The listing builds one solid part. Answer for the finished solid, in the listing's coordinates (mm). A direction names the side the tool comes from. Coordinates: 2 decimals unless noted, no trailing zeros. Write each loop counter-clockwise with the first axis right and the second up, starting at its lowest first coordinate (ties: lowest second). Pieces come first, ordered by that corner, then holes.
(1) Straight lines are drawn through the part: line 1 (X direction, y = -2.5, z = -21.5); line 2 (X direction, y = -17, z = 30.5); line 3 (Z direction, x = 26, y = -11). For each, find the intervals that lie inside material, in ascending order.
(2) The part is cut by section A-A on y = -11. Determine the outline of the cut face in (x, z).
(3) The part is cut by section D-D on z = 13. Determine the outline of the cut face in (x, y), plus the area to 3 significant figures.
(4) The part is cut by section C-C on z = 32.5. Determine the outline of the cut face in (x, y), plus the area to 3 significant figures.
(5) The part is cut by section B-B on x = 11.5. Determine the outline of the cut face in (y, z), plus the area to 3 significant figures.
(6) Which of the six approach directions +Z, -Z, +X, -X, +Y, -Y give full straight-line access (tool end or side, diameter ignored) to faces 1 (the cylindrical face through (4.888, 3.402, 28.834)), 2 (the cylindrical face through (9.86, 1.43, 45.14)), 3 (the flat face through (23, -8, 16)), 4 (the cylindrical face through (26.41, 9.71, 57.75))?
(7) For a pull along Y with two mould halves and no side action, classify faces 5 (the flat face through (23, 7, -28.402)), 6 (the cylindrical face through (-2.43, 23.376, 15.517)), 7 (the cylindrical face through (-1.479, -3.464, 33.028)) as +Y half, -Y half, draft (parallel to the pull), parting line (faces both ways), or undercut.
(8) Given P1, Ø1.5, axis at x = 16.5, z = 42.5, coming from the -Y side; P2, Ø6, axis at x = 24, z = 42, coming from the +Y side; P3, Ø10, axis at x = 11, z = 26.5, coming from the -Y side, each flat-ended and moving along its own axis, determine where each tip first touches the part or whether it passes through.
from build123d import *

# Parameters (mm, degrees)
RESSALTO_EXTRUS_O2_DEPTH      = 30
RESSALTO_EXTRUS_O3_DEPTH      = 3
RESSALTO_EXTRUS_O4_DEPTH      = 3
RESSALTO_EXTRUS_O4_DEPTH_BACK = 10
CORTE_EXTRUS_O1_DEPTH         = 10
CORTE_EXTRUS_O2_DEPTH         = 23.75
ESBO_O10_R                    = 1.5
CORTE_EXTRUS_O3_DEPTH         = 10
CORTE_EXTRUS_O4_DEPTH         = 10
FILETE2_R                     = 2
ESBO_O13_R                    = 1.5
CORTE_EXTRUS_O5_DEPTH         = 16
CORTE_EXTRUS_O11_DEPTH        = 117
FILETE7_R                     = 6
ESBO_O18_R                    = 4
CORTE_EXTRUS_O13_DEPTH        = 22
ESBO_O19_R                    = 4
CORTE_EXTRUS_O14_DEPTH        = 22


with BuildPart() as part:
    # Esboço2 → Ressalto-extrusão2 (new body)
    with BuildSketch(Plane(origin=(0, 0, 0), x_dir=(0, 0, -1), z_dir=(1, 0, 0))):
        with BuildLine():
            Line((2.90159992, -0.062465938), (-35.09840008, -0.062465938))
            Line((-35.09840008, -0.062465938), (-39.886084903, -0.062465938))
            ThreePointArc((-39.886084903, -0.062465938), (-45.202180234, 1.467638524), (-48.891439328, 5.589707975))
            ThreePointArc((-48.891439328, 5.589707975), (-52.096536948, 9.772081499), (-56.69840008, 12.338743681))
            ThreePointArc((-56.69840008, 12.338743681), (-59.373224015, 11.895603401), (-60.59840008, 9.476926077))
            Line((-60.59840008, 9.476926077), (-60.59840008, 20.976926077))
            ThreePointArc((-60.59840008, 20.976926077), (-59.719720424, 23.09824642), (-57.59840008, 23.976926077))
            Line((-57.59840008, 23.976926077), (25.40159992, 23.976926077))
            ThreePointArc((25.40159992, 23.976926077), (27.522920263, 23.09824642), (28.40159992, 20.976926077))
            Line((28.40159992, 20.976926077), (28.40159992, 9.476926077))
            ThreePointArc((28.40159992, 9.476926077), (27.176423855, 11.895603401), (24.50159992, 12.338743681))
            ThreePointArc((24.50159992, 12.338743681), (19.899736788, 9.772081499), (16.694639168, 5.589707975))
            ThreePointArc((16.694639168, 5.589707975), (13.005380073, 1.467638524), (7.689284743, -0.062465938))
            Line((7.689284743, -0.062465938), (2.90159992, -0.062465938))
        make_face()
    extrude(amount=RESSALTO_EXTRUS_O2_DEPTH)

    # Esboço3 → Ressalto-extrusão3 (add)
    with BuildSketch(Plane.ZY):
        with BuildLine():
            Line((60.59840008, 15.226926077), (60.59840008, 20.976926077))
            ThreePointArc((60.59840008, 20.976926077), (59.719720424, 23.09824642), (57.59840008, 23.976926077))
            Line((57.59840008, 23.976926077), (16.09840008, 23.976926077))
            Line((16.09840008, 23.976926077), (-25.40159992, 23.976926077))
            ThreePointArc((-25.40159992, 23.976926077), (-27.522920263, 23.09824642), (-28.40159992, 20.976926077))
            Line((-28.40159992, 20.976926077), (-28.40159992, 15.226926077))
            Line((-28.40159992, 15.226926077), (-28.40159992, -16.773073923))
            ThreePointArc((-28.40159992, -16.773073923), (-27.522920263, -18.894394267), (-25.40159992, -19.773073923))
            Line((-25.40159992, -19.773073923), (57.59840008, -19.773073923))
            ThreePointArc((57.59840008, -19.773073923), (59.719720424, -18.894394267), (60.59840008, -16.773073923))
            Line((60.59840008, -16.773073923), (60.59840008, 15.226926077))
        make_face()
    extrude(amount=RESSALTO_EXTRUS_O3_DEPTH)

    # Esboço4 → Ressalto-extrusão4 (add, two sides)
    with BuildSketch(Plane(origin=(30, 0, 0), x_dir=(0, 0, -1), z_dir=(1, 0, 0))) as ressalto_extrus_o4_sk:
        with BuildLine():
            Line((-16.09840008, 23.976926077), (25.40159992, 23.976926077))
            ThreePointArc((25.40159992, 23.976926077), (27.522920263, 23.09824642), (28.40159992, 20.976926077))
            Line((28.40159992, 20.976926077), (28.40159992, 15.226926077))
            Line((28.40159992, 15.226926077), (28.40159992, -16.773073923))
            ThreePointArc((28.40159992, -16.773073923), (27.522920263, -18.894394267), (25.40159992, -19.773073923))
            Line((25.40159992, -19.773073923), (-57.59840008, -19.773073923))
            ThreePointArc((-57.59840008, -19.773073923), (-59.719720424, -18.894394267), (-60.59840008, -16.773073923))
            Line((-60.59840008, -16.773073923), (-60.59840008, 15.226926077))
            Line((-60.59840008, 15.226926077), (-60.59840008, 20.976926077))
            ThreePointArc((-60.59840008, 20.976926077), (-59.719720424, 23.09824642), (-57.59840008, 23.976926077))
            Line((-57.59840008, 23.976926077), (-16.09840008, 23.976926077))
        make_face()
    extrude(amount=RESSALTO_EXTRUS_O4_DEPTH)
    extrude(ressalto_extrus_o4_sk.sketch, amount=-RESSALTO_EXTRUS_O4_DEPTH_BACK)

    # Esboço8 → Corte-extrusão1 (cut)
    with BuildSketch(Plane(origin=(33, 0, 0), x_dir=(0, 0, -1), z_dir=(1, 0, 0))):
        with BuildLine():
            Line((-43.59840008, 3.976926077), (11.40159992, 3.976926077))
            ThreePointArc((11.40159992, 3.976926077), (12.815813482, 3.391139639), (13.40159992, 1.976926077))
            Line((13.40159992, 1.976926077), (13.40159992, -7.773073923))
            Line((13.40159992, -7.773073923), (13.40159992, -19.773073923))
            Line((13.40159992, -19.773073923), (-45.59840008, -19.773073923))
            Line((-45.59840008, -19.773073923), (-45.59840008, -7.773073923))
            Line((-45.59840008, -7.773073923), (-45.59840008, 1.976926077))
            ThreePointArc((-45.59840008, 1.976926077), (-45.012613643, 3.391139639), (-43.59840008, 3.976926077))
        make_face()
    extrude(amount=-CORTE_EXTRUS_O1_DEPTH, mode=Mode.SUBTRACT)

    # Esboço9 → Corte-extrusão2 (cut)
    with BuildSketch(Plane(origin=(0, -19.773073923, 0), x_dir=(-1, 0, 0), z_dir=(0, -1, 0))):
        with BuildLine():
            Line((-25, 13.40159992), (-28, 13.40159992))
            ThreePointArc((-28, 13.40159992), (-29.414213562, 12.815813482), (-30, 11.40159992))
            Line((-30, 11.40159992), (-30, -43.59840008))
            ThreePointArc((-30, -43.59840008), (-29.414213562, -45.012613643), (-28, -45.59840008))
            Line((-28, -45.59840008), (-25, -45.59840008))
            ThreePointArc((-25, -45.59840008), (-23.585786438, -45.012613643), (-23, -43.59840008))
            Line((-23, -43.59840008), (-23, 11.40159992))
            ThreePointArc((-23, 11.40159992), (-23.585786438, 12.815813482), (-25, 13.40159992))
        make_face()
    extrude(amount=-CORTE_EXTRUS_O2_DEPTH, mode=Mode.SUBTRACT)

    # Esboço10 → Corte-extrusão3 (cut)
    with BuildSketch(Plane(origin=(0, 0, 0), x_dir=(0, 0, -1), z_dir=(1, 0, 0))):
        with Locations((-55.59840008, 6.338743681)):
            Circle(ESBO_O10_R)
        with Locations((23.40159992, 6.338743681)):
            Circle(ESBO_O10_R)
        with Locations((-16.09840008, -8.562465938)):
            Circle(ESBO_O10_R)
    extrude(amount=-CORTE_EXTRUS_O3_DEPTH, mode=Mode.SUBTRACT)

    # Esboço12 → Corte-extrusão4 (cut)
    with BuildSketch(Plane(origin=(0, 0, 0), x_dir=(0, 0, -1), z_dir=(1, 0, 0))):
        with BuildLine():
            Line((-31.59840008, -2.862465938), (-25.59840008, -2.862465938))
            ThreePointArc((-25.59840008, -2.862465938), (-24.184186518, -3.448252375), (-23.59840008, -4.862465938))
            Line((-23.59840008, -4.862465938), (-23.59840008, -14.773073923))
            ThreePointArc((-23.59840008, -14.773073923), (-24.184186518, -16.187287486), (-25.59840008, -16.773073923))
            Line((-25.59840008, -16.773073923), (-31.59840008, -16.773073923))
            ThreePointArc((-31.59840008, -16.773073923), (-33.012613643, -16.187287486), (-33.59840008, -14.773073923))
            Line((-33.59840008, -14.773073923), (-33.59840008, -4.862465938))
            ThreePointArc((-33.59840008, -4.862465938), (-33.012613643, -3.448252375), (-31.59840008, -2.862465938))
        make_face()
        with BuildLine():
            Line((-6.59840008, -2.862465938), (-0.59840008, -2.862465938))
            ThreePointArc((-0.59840008, -2.862465938), (0.815813482, -3.448252375), (1.40159992, -4.862465938))
            Line((1.40159992, -4.862465938), (1.40159992, -14.773073923))
            ThreePointArc((1.40159992, -14.773073923), (0.815813482, -16.187287486), (-0.59840008, -16.773073923))
            Line((-0.59840008, -16.773073923), (-6.59840008, -16.773073923))
            ThreePointArc((-6.59840008, -16.773073923), (-8.012613643, -16.187287486), (-8.59840008, -14.773073923))
            Line((-8.59840008, -14.773073923), (-8.59840008, -4.862465938))
            ThreePointArc((-8.59840008, -4.862465938), (-8.012613643, -3.448252375), (-6.59840008, -2.862465938))
        make_face()
    extrude(amount=-CORTE_EXTRUS_O4_DEPTH, mode=Mode.SUBTRACT)

    # Filete2
    filete2_edges = [part.edges().sort_by_distance(p)[0] for p in [
        (-3, 2.101926077, 60.59840008),
        (-3, 23.09824642, 59.719720424),
        (-3, 23.976926077, 16.09840008),
        (-3, 23.09824642, -27.522920263),
        (-3, 2.101926077, -28.40159992),
        (-3, -18.894394267, -27.522920263),
        (-3, -19.773073923, 16.09840008),
        (-3, -18.894394267, 59.719720424),
    ]]
    fillet(filete2_edges, radius=FILETE2_R)

    # Esboço13 → Corte-extrusão5 (cut)
    with BuildSketch(Plane.ZY.offset(3)):
        with Locations((27.44840008, 3.976926077)):
            Circle(ESBO_O13_R)
        with Locations((4.74840008, 3.976926077)):
            Circle(ESBO_O13_R)
    extrude(amount=-CORTE_EXTRUS_O5_DEPTH, mode=Mode.SUBTRACT)

    # Esboço16 → Corte-extrusão11 (cut)
    with BuildSketch(Plane(origin=(0, 0, -38.40159992), x_dir=(-1, 0, 0), z_dir=(0, 0, -1))):
        Polygon((-13, 23.976926077), (-33, 11.226201247), (-33, 23.976926077), align=None)
    extrude(amount=-CORTE_EXTRUS_O11_DEPTH, mode=Mode.SUBTRACT)

    # Filete7
    filete7_edges = [part.edges().sort_by_distance(p)[0] for p in [
        (33, 11.226201247, 16.09840008),
    ]]
    fillet(filete7_edges, radius=FILETE7_R)

    # Esboço18 → Corte-extrusão13 (cut)
    with BuildSketch(Plane.ZY.offset(-20)):
        with Locations((-23.40159992, 6.338743681)):
            Circle(ESBO_O18_R)
    extrude(amount=-CORTE_EXTRUS_O13_DEPTH, mode=Mode.SUBTRACT)

    # Esboço19 → Corte-extrusão14 (cut)
    with BuildSketch(Plane.ZY.offset(-20)):
        with Locations((55.59840008, 6.338743681)):
            Circle(ESBO_O19_R)
    extrude(amount=-CORTE_EXTRUS_O14_DEPTH, mode=Mode.SUBTRACT)


solid = part.part
Model answer:
1. line 1: x = -3 to 0, 20 to 33
1. line 2: x = -3 to 0, 20 to 23
1. line 3: z = -28.4 to -13.4, 45.6 to 60.6
2. outline: (-3, -26.4) arc R2 ccw to (-1, -28.4) - (0, -28.4) - (0, -1.4) - (-3, -1.4) - close; (-3, 8.6) - (0, 8.6) - (0, 23.6) - (-3, 23.6) - close; (-3, 33.6) - (0, 33.6) - (0, 60.6) - (-1, 60.6) arc R2 ccw to (-3, 58.6) - close; (20, -28.4) - (33, -28.4) - (33, -13.4) - (23, -13.4) - (23, 45.6) - (33, 45.6) - (33, 60.6) - (20, 60.6) - close
3. outline: (-3, -17.77) arc R2 ccw to (-1, -19.77) - (0, -19.77) - (0, -0.06) - (20, -0.06) - (20, -19.77) - (23, -19.77) - (23, 3.98) - (33, 3.98) - (33, 7.94) arc R6 ccw to (30.23, 13) - (13, 23.98) - (-1, 23.98) arc R2 ccw to (-3, 21.98) - close
3. area: 812 mm2
4. outline: (-3, -17.77) arc R2 ccw to (-1, -19.77) - (0, -19.77) - (0, -16.56) - (-3, -16.56) - close; (-3, -3.08) - (0, -3.08) - (0, -0.06) - (20, -0.06) - (20, -19.77) - (23, -19.77) - (23, 3.98) - (33, 3.98) - (33, 7.94) arc R6 ccw to (30.23, 13) - (13, 23.98) - (-1, 23.98) arc R2 ccw to (-3, 21.98) - close
4. area: 772 mm2
5. outline: (-0.06, -7.69) arc R10 ccw to (5.59, -16.69) arc R13 cw to (12.34, -24.5) arc R3 cw to (9.48, -28.4) - (20.98, -28.4) arc R3 ccw to (23.98, -25.4) - (23.98, 57.6) arc R3 ccw to (20.98, 60.6) - (9.48, 60.6) arc R3 cw to (12.34, 56.7) arc R13 cw to (5.59, 48.89) arc R10 ccw to (-0.06, 39.89) - close; hole circle Ø3 at (3.98, 4.75); hole circle Ø3 at (3.98, 27.45)
5. area: 1,840 mm2
6. face 1: -X
6. face 2: +Z, -Y
6. face 3: +X, -Y
6. face 4: +X
7. face 5: draft
7. face 6: +Y half
7. face 7: undercut
8. P1: stops at y = 0.11
8. P2: stops at y = 18.88
8. P3: stops at y = -0.06
